Input: part model. Units: mm. Frame: model coordinates. Coordinates: 2 decimals unless noted, no trailing zeros. Order: outer loops, then holes, each group sorted by start corner. A loop starts at its lowest first (then second) coordinate and runs counter-clockwise, first axis right, second up. Notation, with made-up numbers: (-5, -27) -> (8, -27) arc R35 ccw to (8, 12) -> close; hole circle Ø8 at (67.25, -1.5). An arc over 180 degrees is marked (long way). One line per question, with ' | ' between items.
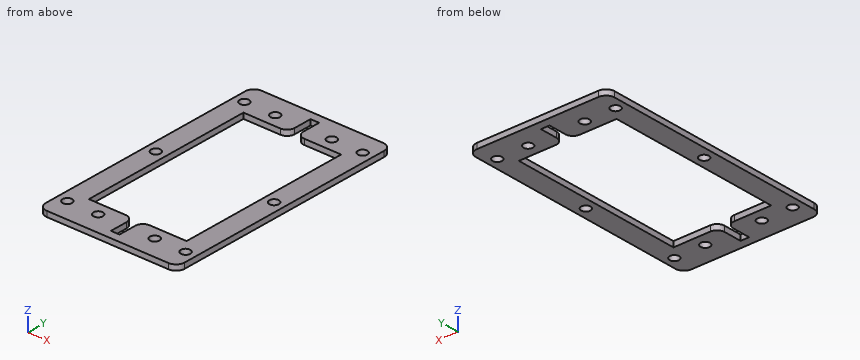
```python
from build123d import *

# Parameters (mm, degrees)
F0_R     = 2.75
F1_DEPTH = 3.175


# Not quite as in the source:
# - a length typed as a fraction of an inch, garbled in the dataset ("3 / 203.2 mm" for 3/8 in), is restored


with BuildPart() as f1:
    # F0 (on Top) → F1 (new body)
    with BuildSketch(Plane.XY):
        with BuildLine():
            Line((-35.5, -71.5), (35.5, -71.5))
            ThreePointArc((35.5, -71.5), (39.0355339059, -70.0355339059), (40.5, -66.5))
            Line((40.5, -66.5), (40.5, 66.5))
            ThreePointArc((40.5, 66.5), (39.0355339059, 70.0355339059), (35.5, 71.5))
            Line((35.5, 71.5), (-35.5, 71.5))
            ThreePointArc((-35.5, 71.5), (-39.0355339059, 70.0355339059), (-40.5, 66.5))
            Line((-40.5, 66.5), (-40.5, -66.5))
            ThreePointArc((-40.5, -66.5), (-39.0355339059, -70.0355339059), (-35.5, -71.5))
        make_face()
        with Locations((-34.5, -59)):
            Circle(F0_R, mode=Mode.SUBTRACT)
        with Locations((-16.5, -59)):
            Circle(F0_R, mode=Mode.SUBTRACT)
        with Locations((16.5, -59)):
            Circle(F0_R, mode=Mode.SUBTRACT)
        with Locations((34.5, -59)):
            Circle(F0_R, mode=Mode.SUBTRACT)
        with Locations((-34.5, 0)):
            Circle(F0_R, mode=Mode.SUBTRACT)
        with Locations((-34.5, 59)):
            Circle(F0_R, mode=Mode.SUBTRACT)
        with Locations((-16.5, 59)):
            Circle(F0_R, mode=Mode.SUBTRACT)
        with BuildLine():
            Line((28.5, 51.5), (28.5, -51.5))
            Line((28.5, -51.5), (7, -51.5))
            ThreePointArc((7, -51.5), (3.8180194847, -52.8180194847), (2.5, -56))
            Line((2.5, -56), (2.5, -66.5))
            Line((2.5, -66.5), (-2.5, -66.5))
            Line((-2.5, -66.5), (-2.5, -56))
            ThreePointArc((-2.5, -56), (-3.8180194847, -52.8180194847), (-7, -51.5))
            Line((-7, -51.5), (-28.5, -51.5))
            Line((-28.5, -51.5), (-28.5, 51.5))
            Line((-28.5, 51.5), (-7, 51.5))
            ThreePointArc((-7, 51.5), (-3.8180194847, 52.8180194847), (-2.5, 56))
            Line((-2.5, 56), (-2.5, 66.5))
            Line((-2.5, 66.5), (2.5, 66.5))
            Line((2.5, 66.5), (2.5, 56))
            ThreePointArc((2.5, 56), (3.8180194847, 52.8180194847), (7, 51.5))
            Line((7, 51.5), (28.5, 51.5))
        make_face(mode=Mode.SUBTRACT)
        with Locations((34.5, 0)):
            Circle(F0_R, mode=Mode.SUBTRACT)
        with Locations((16.5, 59)):
            Circle(F0_R, mode=Mode.SUBTRACT)
        with Locations((34.5, 59)):
            Circle(F0_R, mode=Mode.SUBTRACT)
    extrude(amount=F1_DEPTH)


solid = f1.part
```
1. Cut plane A-A, the plane x = -16.5. Return loops of the section in (y, z) (3 decimals).
Recorded:
outline: (-71.5, 0) -> (-61.75, 0) -> (-61.75, 3.175) -> (-71.5, 3.175) -> close; (-56.25, 0) -> (-51.5, 0) -> (-51.5, 3.175) -> (-56.25, 3.175) -> close; (51.5, 0) -> (56.25, 0) -> (56.25, 3.175) -> (51.5, 3.175) -> close; (61.75, 0) -> (71.5, 0) -> (71.5, 3.175) -> (61.75, 3.175) -> close
2. Ray query, line 1 (Y direction, x = 34.5, z = 0.75); line 2 (Y direction, x = -16.5, z = 0.85); line 3 (X direction, y = 20, z = 0.9). Return the intervals inside material, ascending. Write a range as [from, to].
Recorded:
line 1: y = [-71.5, -61.75], [-56.25, -2.75], [2.75, 56.25], [61.75, 71.5] | line 2: y = [-71.5, -61.75], [-56.25, -51.5], [51.5, 56.25], [61.75, 71.5] | line 3: x = [-40.5, -28.5], [28.5, 40.5]
3. Cut plane B-B, the plane y = -10.5. Return loops of the section in (x, z) (3 decimals).
Recorded:
outline: (-40.5, 0) -> (-28.5, 0) -> (-28.5, 3.175) -> (-40.5, 3.175) -> close; (28.5, 0) -> (40.5, 0) -> (40.5, 3.175) -> (28.5, 3.175) -> close
4. Cut plane C-C, the plane z = 2.55. State how many separate pieces and enclosed holes the cut face has, and give its area (3 significant figures).
Recorded:
separate pieces: 1 | enclosed holes: 11 | area: 5,290 mm^2
5. Cut plane D-D, the plane y = -59. Return loops of the section in (x, z) (3 decimals), and give its area (3 significant figures).
Recorded:
outline: (-40.5, 0) -> (-37.25, 0) -> (-37.25, 3.175) -> (-40.5, 3.175) -> close; (-31.75, 0) -> (-19.25, 0) -> (-19.25, 3.175) -> (-31.75, 3.175) -> close; (-13.75, 0) -> (-2.5, 0) -> (-2.5, 3.175) -> (-13.75, 3.175) -> close; (2.5, 0) -> (13.75, 0) -> (13.75, 3.175) -> (2.5, 3.175) -> close; (19.25, 0) -> (31.75, 0) -> (31.75, 3.175) -> (19.25, 3.175) -> close; (37.25, 0) -> (40.5, 0) -> (40.5, 3.175) -> (37.25, 3.175) -> close | area: 171 mm^2
